```python
from build123d import *

# Parameters (mm, degrees)
CYLINDER1525_R               = 1.5
CYLINDER1525_DEPTH           = 50
CYLINDER1525_PLACEMENT_ANGLE = 45
CYLINDER1508_R               = 1.5
CYLINDER1508_DEPTH           = 50
CYLINDER1508_PLACEMENT_ANGLE = 135
CYLINDER1511_R               = 1.5
CYLINDER1511_DEPTH           = 50
CYLINDER1521_R               = 1.5
CYLINDER1521_DEPTH           = 50
CYLINDER1521_PLACEMENT_ANGLE = 225
CYLINDER1514_R               = 1.5
CYLINDER1514_DEPTH           = 50
CYLINDER1505_R               = 1.5
CYLINDER1505_DEPTH           = 50
CYLINDER1505_PLACEMENT_ANGLE = 45
CYLINDER1519_R               = 1.5
CYLINDER1519_DEPTH           = 50
CYLINDER1516_R               = 52
CYLINDER1516_DEPTH           = 16
BOX524_W                     = 108
BOX524_H                     = 36
BOX524_DEPTH                 = 12


with BuildPart() as obj1:
    # Cylinder1525 → Cylinder1525 (new body)
    with BuildSketch(Plane.XY):
        Circle(CYLINDER1525_R)
    extrude(amount=CYLINDER1525_DEPTH)


with BuildPart() as obj1_1:
    # Cylinder1525 placement: moved
    add(obj1.part.moved(Location((39.59798, -39.59798, 2))).rotate(Axis((39.59798, -39.59798, 2), (0, 0, 1)), CYLINDER1525_PLACEMENT_ANGLE))


with BuildPart() as obj2:
    # Cylinder1508 → Cylinder1508 (new body)
    with BuildSketch(Plane.XY):
        Circle(CYLINDER1508_R)
    extrude(amount=CYLINDER1508_DEPTH)


with BuildPart() as obj2_1:
    # Cylinder1508 placement: moved
    add(obj2.part.moved(Location((39.59798, 39.59798, 2))).rotate(Axis((39.59798, 39.59798, 2), (0, 0, 1)), CYLINDER1508_PLACEMENT_ANGLE))


with BuildPart() as obj3:
    # Cylinder1511 → Cylinder1511 (new body)
    with BuildSketch(Plane(origin=(0, 56, 2), x_dir=(-1, 0, 0), z_dir=(0, 0, 1))):
        Circle(CYLINDER1511_R)
    extrude(amount=CYLINDER1511_DEPTH)


with BuildPart() as obj4:
    # Cylinder1521 → Cylinder1521 (new body)
    with BuildSketch(Plane.XY):
        Circle(CYLINDER1521_R)
    extrude(amount=CYLINDER1521_DEPTH)


with BuildPart() as obj4_1:
    # Cylinder1521 placement: moved
    add(obj4.part.moved(Location((-39.59798, 39.59798, 2))).rotate(Axis((-39.59798, 39.59798, 2), (0, 0, 1)), CYLINDER1521_PLACEMENT_ANGLE))


with BuildPart() as obj5:
    # Cylinder1514 → Cylinder1514 (new body)
    with BuildSketch(Plane(origin=(-56, 0, 2), x_dir=(0, -1, 0), z_dir=(0, 0, 1))):
        Circle(CYLINDER1514_R)
    extrude(amount=CYLINDER1514_DEPTH)


with BuildPart() as obj6:
    # Cylinder1505 → Cylinder1505 (new body)
    with BuildSketch(Plane.XY):
        Circle(CYLINDER1505_R)
    extrude(amount=CYLINDER1505_DEPTH)


with BuildPart() as obj6_1:
    # Cylinder1505 placement: moved
    add(obj6.part.moved(Location((-39.59798, -39.59798, 2))).rotate(Axis((-39.59798, -39.59798, 2), (0, 0, -1)), CYLINDER1505_PLACEMENT_ANGLE))


with BuildPart() as compound908:
    # Cylinder1519 → Cylinder1519 (new body)
    with BuildSketch(Plane(origin=(0, -56, 2), x_dir=(1, 0, 0), z_dir=(0, 0, 1))):
        Circle(CYLINDER1519_R)
    extrude(amount=CYLINDER1519_DEPTH)

    # Compound908: union obj1, obj2, obj3, obj4, obj5, obj6
    add(obj1_1.part)
    add(obj2_1.part)
    add(obj3.part)
    add(obj4_1.part)
    add(obj5.part)
    add(obj6_1.part)


with BuildPart() as obj7:
    # Cylinder1516 → Cylinder1516 (new body)
    with BuildSketch(Plane.XY.offset(20)):
        Circle(CYLINDER1516_R)
    extrude(amount=CYLINDER1516_DEPTH)


with BuildPart() as cut559:
    # Box524 → Box524 (new body)
    with BuildSketch(Plane(origin=(-54, -53, 20), x_dir=(1, 0, 0), z_dir=(0, 0, 1))):
        with Locations((54, 18)):
            Rectangle(BOX524_W, BOX524_H)
    extrude(amount=BOX524_DEPTH)

    # Cut550: cut obj7
    add(obj7.part, mode=Mode.SUBTRACT)


with BuildPart() as cut559_1:
    # Cut550 placement: moved
    add(cut559.part.moved(Location((0, 0, -10))))

    # Cut559: cut Compound908
    add(compound908.part, mode=Mode.SUBTRACT)


with BuildPart() as cut559_2:
    # Cut559 placement: moved
    add(cut559_1.part.moved(Location((0, 0, -4))))


solid = cut559_2.part
```
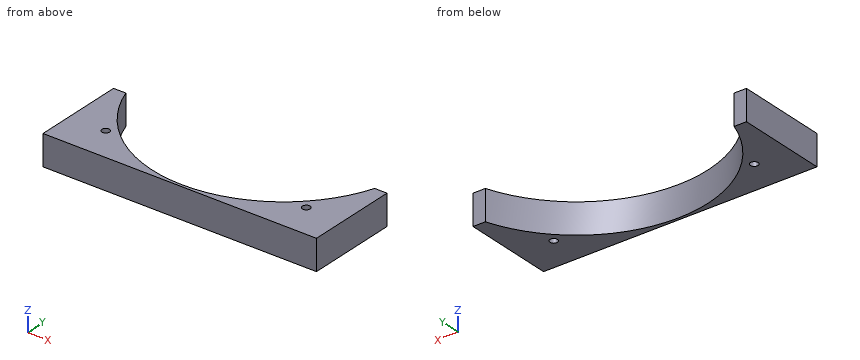
Geometry: final body of the model. Coordinates: model frame, mm. Coordinates: 2 decimals unless noted, no trailing zeros. Order: outer loops, then holes, each group sorted by start corner. A loop starts at its lowest first (then second) coordinate and runs counter-clockwise, first axis right, second up. Notation, with made-up numbers: (56.5, 43.25) -> (65.5, 43.25) arc R28 cw to (65.5, 79.25) -> close; hole circle Ø2 at (7, 52.25). An arc over 180 degrees is marked (long way). Answer in a Markdown table with one row per item.
Item 1: Section A-A on y = -50. Output: boundary loops of the cut face in (x, z).
Return value:
| item | result |
|---|---|
| outline | (-54, 6) -> (-14.28, 6) -> (-14.28, 18) -> (-54, 18) -> close; (14.28, 6) -> (54, 6) -> (54, 18) -> (14.28, 18) -> close |
Item 2: Section B-B on z = 11.75. Output: boundary loops of the cut face in (x, y), plus the area to 3 significant figures.
Return value:
| item | result |
|---|---|
| outline | (-54, -53) -> (54, -53) -> (54, -17) -> (49.14, -17) arc R52 cw to (-49.14, -17) -> (-54, -17) -> close; hole circle Ø3 at (-39.6, -39.6); hole circle Ø3 at (39.6, -39.6) |
| area | 1,360 mm² |
Item 3: Section D-D on x = -17. Output: boundary loops of the cut face in (y, z).
Return value:
| item | result |
|---|---|
| outline | (-53, 6) -> (-49.14, 6) -> (-49.14, 18) -> (-53, 18) -> close |
Item 4: Contact query for a flat-ended pin moving along its axis: P1, Ø3, axis at x = -10, z = 16, coming from the +Y side. Output: stop coordinate, or through.
Return value:
| item | result |
|---|---|
| P1 | stops at y = -50.71 |
Item 5: Section C-C on y = -34. Output: boundary loops of the cut face in (x, z), plus the area to 3 significant figures.
Return value:
| item | result |
|---|---|
| outline | (-54, 6) -> (-39.34, 6) -> (-39.34, 18) -> (-54, 18) -> close; (39.34, 6) -> (54, 6) -> (54, 18) -> (39.34, 18) -> close |
| area | 352 mm² |
Item 6: Ray query, L1, parallel to X at y = -39.5, z = 17.75; L2, parallel to X at y = -38.5, z = 15.75; L3, parallel to X at y = -34, z = 12.5. Return the intervals inside material, ascending.
Return value:
| item | result |
|---|---|
| L1 | x = -54 to -41.09, -38.1 to -33.82, 33.82 to 38.1, 41.09 to 54 |
| L2 | x = -54 to -40.62, -38.58 to -34.95, 34.95 to 38.58, 40.62 to 54 |
| L3 | x = -54 to -39.34, 39.34 to 54 |
